Geometry: see drawing. Coordinates: mm, zero at the bounding-box minimum. Coordinates: 2 decimals unless noted, no trailing zeros. Write each loop counter-clockwise with the first axis right and the second up, starting at its lowest first coordinate (ties: lowest second). Pieces come first, ordered by that corner, then holes. Notation, with made-up numbers: M -38,33 L -3,33 A30 ccw -3,63 Z; hole C 57.25,28 d6. An arc over 180 degrees is marked long. Write item = value, one per line. Start each with the question number.
1. Pin query (flat end, axial travel): pin 1 Ø3 at (y, z) = (19.85, 3.39) entering from +X (1 decimal); pin 2 Ø6 at (x, z) = (10, 14.5) entering from +Y (1 decimal); pin 3 Ø2.5 at (x, y) = (9.5, 1) entering from +Z. Return the tip coordinate at first contact, or that it passes through.
2. Section query D-D (x = 1.5). Output: boundary loops of the cut face in (y, z) (1 decimal).
3. Section query B-B (y = 24.5). Output: boundary loops of the cut face in (x, z) (1 decimal).
4. Line query: line 1 along X through (y, z) = (11, 26) (1 decimal); line 2 along Y through (x, z) = (2, 9.5) (1 decimal). Output: solid intervals per line, ascending.
5. Section query C-C (z = 2.5). Output: boundary loops of the cut face in (x, y) (1 decimal).
6. Section query A-A (z = 27). Output: boundary loops of the cut face in (x, y) (1 decimal).
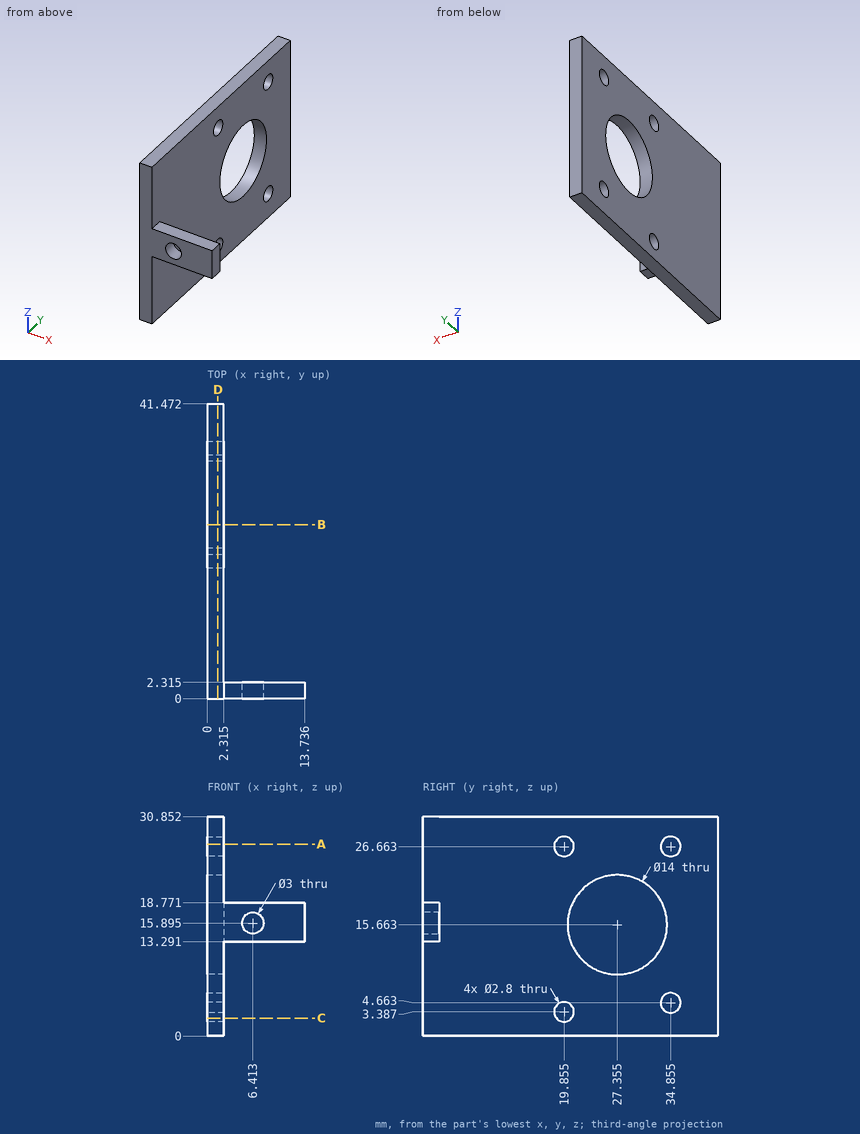
Results are:
q1.pin_1 = 2.3
q1.pin_2 = 2.3
q1.pin_3 = 18.77
q2.outline = M 0,0 L 41.5,0 L 41.5,30.9 L 0,30.9 Z; hole C 19.9,3.4 d2.8; hole C 19.9,26.7 d2.8; hole C 27.4,15.7 d14; hole C 34.9,4.7 d2.8; hole C 34.9,26.7 d2.8
q3.outline = M 0,0 L 2.3,0 L 2.3,9.3 L 0,9.3 Z; M 0,22.1 L 2.3,22.1 L 2.3,30.9 L 0,30.9 Z
q4.line_1 = 0 to 2.3
q4.line_2 = 0 to 24, 30.7 to 41.5
q5.outline = M 0,0 L 2.3,0 L 2.3,18.8 L 0,18.8 Z; M 0,20.9 L 2.3,20.9 L 2.3,41.5 L 0,41.5 Z
q6.outline = M 0,0 L 2.3,0 L 2.3,18.5 L 0,18.5 Z; M 0,21.2 L 2.3,21.2 L 2.3,33.5 L 0,33.5 Z; M 0,36.2 L 2.3,36.2 L 2.3,41.5 L 0,41.5 Z
